Source: CAD feature listing. Evaluate the final solid. Frame: model axes, mm. Face numbers are marked on the shaded views. A direction names the side the tool comes from. Coordinates: 2 decimals unless noted, no trailing zeros. Write each loop counter-clockwise with the first axis right and the second up, starting at its lowest first coordinate (ties: lowest second). Pieces come first, ordered by that corner, then holes. Notation, with made-up numbers: (-32.75, 56.5) - (-19.75, 56.5) arc R27 ccw to (-19.75, 84.5) - close; hole circle Ø1 at (31.25, 29). An arc over 180 degrees is marked (long way). One line per question, with ' | ' between items. Start each with the question number.
Q1. Cut plane B-B, the plane x = 63. Return loops of the section in (y, z) (1 decimal), plus the area to 3 significant figures.
Q2. Cut plane C-C, the plane x = -86. Return loops of the section in (y, z) (1 decimal).
Q3. Access query for the marked faces 1 and 2. Directions: +Z, -Z, +X, -X, +Y, -Y. A direction counts if a zero-diameter tool reaches every point of the face in a straight line with its end or side. Return the directions, or none.
Q4. Line query: line 1 (X direction, y = 24, z = -16.5) (3 decimals); line 2 (X direction, y = -9, z = -23.5); line 3 (X direction, y = 52.5, z = 10.5). Output: solid intervals per line, ascending.
Q5. Draft query along X for the marked faces 3, 4 and 5. Return one class per face: +X half, -X half, draft (parallel to the pull), parting line (faces both ways), or undercut.
Q6. Contact query for flat-ended pins moving along their axis: P1, Ø3, axis at y = 37, z = -12.5, coming from the -X side; P2, Ø5, axis at x = 123, z = 17, coming from the -Y side; P3, Ø1.5, axis at x = 40, z = 20, coming from the +Y side; P4, Ø6, axis at x = -56.5, z = -6.5, coming from the +Y side. Output: stop coordinate, or through.
```python
from build123d import *

# Parameters (mm, degrees)
SKETCH1_R               = 20.6375
BOSS_EXTRUDE1_DEPTH     = 9.525
SKETCH2_R               = 20.6375
BOSS_EXTRUDE3_DEPTH     = 15.875
SKETCH3_R               = 15.631220112
BOSS_EXTRUDE4_DEPTH     = 15.875
CUT_EXTRUDE1_DEPTH      = 85.544622325
CUT_EXTRUDE1_DEPTH_BACK = 85.544622325
CUT_EXTRUDE2_DEPTH      = 85.544622414
CUT_EXTRUDE2_DEPTH_BACK = 85.544622414
SKETCH6_R               = 17.4625
BOSS_EXTRUDE5_DEPTH     = 127
BOSS_EXTRUDE6_START     = 127
SKETCH7_R               = 17.4625
BOSS_EXTRUDE6_DEPTH     = 127


with BuildPart() as part:
    # Sketch1 → Boss-Extrude1 (new body)
    # profile 1 of 2: a face of its own
    with BuildSketch(Plane(origin=(0, 0, 0), x_dir=(0, 0, -1), z_dir=(1, 0, 0))):
        with BuildLine():
            ThreePointArc((22.225, 53.18125), (0, 75.40625), (-22.225, 53.18125))
            Line((-22.225, 53.18125), (-27.771661542, 6.727959587))
            Line((-27.771661542, 6.727959587), (-28.575, 0))
            ThreePointArc((-28.575, 0), (0, -28.575), (28.575, 0))
            Line((28.575, 0), (27.771661542, 6.727959587))
            Line((27.771661542, 6.727959587), (22.225, 53.18125))
        make_face()
        Circle(SKETCH1_R, mode=Mode.SUBTRACT)
    # profile 2 of 2: a face of its own
    with BuildSketch(Plane(origin=(0, 0, 0), x_dir=(0, 0, -1), z_dir=(1, 0, 0))):
        Circle(SKETCH1_R)
    extrude(amount=BOSS_EXTRUDE1_DEPTH)

    # Sketch2 → Boss-Extrude3 (add)
    with BuildSketch(Plane.ZY):
        Circle(SKETCH2_R)
    extrude(amount=BOSS_EXTRUDE3_DEPTH)

    # Sketch3 → Boss-Extrude4 (add)
    with BuildSketch(Plane(origin=(9.525, 0, 0), x_dir=(0, 0, -1), z_dir=(1, 0, 0))):
        with Locations((0, 53.18125)):
            Circle(SKETCH3_R)
    extrude(amount=BOSS_EXTRUDE4_DEPTH)

    # Sketch4 → Cut-Extrude1 (cut, two sides: drawn at the far end of the back side and taken through both)
    with BuildSketch(Plane.XY.offset(-CUT_EXTRUDE1_DEPTH_BACK)):
        with BuildLine():
            Line((4.7625, 75.40625), (-6.178104272, 75.40625))
            Line((-6.178104272, 75.40625), (-6.178104272, 53.18125))
            Line((-6.178104272, 53.18125), (0, 53.18125))
            ThreePointArc((0, 53.18125), (0.936646322, 64.603307931), (4.7625, 75.40625))
        make_face()
    extrude(amount=CUT_EXTRUDE1_DEPTH + CUT_EXTRUDE1_DEPTH_BACK, mode=Mode.SUBTRACT)

    # Sketch5 → Cut-Extrude2 (cut, two sides: drawn at the far end of the back side and taken through both)
    with BuildSketch(Plane.XY.offset(-CUT_EXTRUDE2_DEPTH_BACK)):
        with BuildLine():
            Line((4.7625, -28.575), (17.4625, -28.575))
            Line((17.4625, -28.575), (17.4625, 0))
            Line((17.4625, 0), (9.525, 0))
            ThreePointArc((9.525, 0), (8.641404401, -14.537109067), (4.7625, -28.575))
        make_face()
    extrude(amount=CUT_EXTRUDE2_DEPTH + CUT_EXTRUDE2_DEPTH_BACK, mode=Mode.SUBTRACT)

    # Mirror1: part across plane


with BuildPart() as part_1:
    add(part.part)
    add(part.part.mirror(Plane(origin=(25.4, 53.18125, 0), x_dir=(0, 0, 1), z_dir=(1, 0, 0))))

    # Sketch6 → Boss-Extrude5 (add)
    with BuildSketch(Plane.ZY.offset(15.875)):
        Circle(SKETCH6_R)
    extrude(amount=BOSS_EXTRUDE5_DEPTH)

    # Sketch7 → Boss-Extrude6 (add)
    with BuildSketch(Plane(origin=(66.675, 0, 0), x_dir=(0, 0, -1), z_dir=(1, 0, 0)).offset(BOSS_EXTRUDE6_START)):
        with Locations(Location((0, 0, 0), (0, 0, 180))):
            Circle(SKETCH7_R)
    extrude(amount=-BOSS_EXTRUDE6_DEPTH)


solid = part_1.part
```
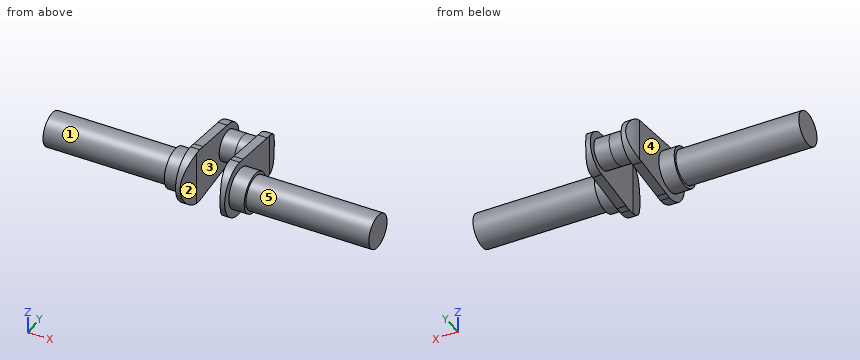
Reply:
1) outline: circle Ø41.3 at (0, 0) | area: 1,340 mm^2
2) outline: circle Ø34.9 at (0, 0)
3) face 1: -X | face 2: +Z, -Z, -Y
4) line 1: x = 0 to 9.525, 41.275 to 50.8 | line 2: x = 0 to 9.34, 41.46 to 50.8 | line 3: x = 0 to 50.8
5) face 3: undercut | face 4: -X half | face 5: draft
6) P1: stops at x = 0 | P2: stops at y = -9.73 | P3: passes through | P4: stops at y = 17.11
